Check sheet for the modelled part. Datum: model origin and axes. Units: mm. Give positions to 0.01 mm unless a question says otherwise; leave off trailing zeros. Order: outer loops, then holes, each group sorted by start corner. A loop starts at its lowest first (then second) coordinate and runs counter-clockwise, first axis right, second up.
```python
from build123d import *

# Parameters (mm, degrees)
ESQUISSE1_R        = 123.074849798
ESQUISSE1_R_2      = 2.953796395
ESQUISSE1_R_3      = 35
ESQUISSE1_R_4      = 3.375
ESQUISSE1_R_5      = 22.5
BOSS_EXTRU_1_DEPTH = 5
CHANFREIN1_SIZE    = 3


with BuildPart() as part:
    # Esquisse1 → Boss.-Extru.1 (new body)
    with BuildSketch(Plane.XY):
        Circle(ESQUISSE1_R)
        with Locations((0, 115.5)):
            Circle(ESQUISSE1_R_2, mode=Mode.SUBTRACT)
        Circle(ESQUISSE1_R_3, mode=Mode.SUBTRACT)
        with Locations((74.241968919, 88.47813318)):
            Circle(ESQUISSE1_R_2, mode=Mode.SUBTRACT)
        with Locations((113.745295473, 20.056364521)):
            Circle(ESQUISSE1_R_2, mode=Mode.SUBTRACT)
        with Locations((100.025934137, -57.75)):
            Circle(ESQUISSE1_R_2, mode=Mode.SUBTRACT)
        with Locations((39.503326554, -108.534497701)):
            Circle(ESQUISSE1_R_2, mode=Mode.SUBTRACT)
        with Locations((-39.503326554, -108.534497701)):
            Circle(ESQUISSE1_R_2, mode=Mode.SUBTRACT)
        with Locations((-100.025934137, -57.75)):
            Circle(ESQUISSE1_R_2, mode=Mode.SUBTRACT)
        with Locations((-113.745295473, 20.056364521)):
            Circle(ESQUISSE1_R_2, mode=Mode.SUBTRACT)
        with Locations((-74.241968919, 88.47813318)):
            Circle(ESQUISSE1_R_2, mode=Mode.SUBTRACT)
        with Locations((0, 50)):
            Circle(ESQUISSE1_R_4, mode=Mode.SUBTRACT)
        with Locations((50, 0)):
            Circle(ESQUISSE1_R_4, mode=Mode.SUBTRACT)
        with Locations((0, -50)):
            Circle(ESQUISSE1_R_4, mode=Mode.SUBTRACT)
        with Locations((-50, 0)):
            Circle(ESQUISSE1_R_4, mode=Mode.SUBTRACT)
        with Locations((0, 82.5)):
            Circle(ESQUISSE1_R_5, mode=Mode.SUBTRACT)
        with Locations((58.336309448, 58.336309448)):
            Circle(ESQUISSE1_R_5, mode=Mode.SUBTRACT)
        with Locations((82.5, 0)):
            Circle(ESQUISSE1_R_5, mode=Mode.SUBTRACT)
        with Locations((58.336309448, -58.336309448)):
            Circle(ESQUISSE1_R_5, mode=Mode.SUBTRACT)
        with Locations((0, -82.5)):
            Circle(ESQUISSE1_R_5, mode=Mode.SUBTRACT)
        with Locations((-58.336309448, -58.336309448)):
            Circle(ESQUISSE1_R_5, mode=Mode.SUBTRACT)
        with Locations((-82.5, 0)):
            Circle(ESQUISSE1_R_5, mode=Mode.SUBTRACT)
        with Locations((-58.336309448, 58.336309448)):
            Circle(ESQUISSE1_R_5, mode=Mode.SUBTRACT)
    extrude(amount=BOSS_EXTRU_1_DEPTH)

    # Chanfrein1
    chanfrein1_edges = [part.edges().sort_by_distance(p)[0] for p in [
        (71.288172524, 88.47813318, 0),
        (110.791499078, 20.056364521, 0),
        (97.072137742, -57.75, 0),
        (36.549530159, -108.534497701, 0),
        (-42.457122949, -108.534497701, 0),
        (-102.979730532, -57.75, 0),
        (-116.699091868, 20.056364521, 0),
        (-77.195765314, 88.47813318, 0),
        (-2.953796395, 115.5, 0),
    ]]
    chamfer(chanfrein1_edges, length=CHANFREIN1_SIZE)


solid = part.part
```
(1) Cross-section at A-A on x = -14. Enter the section's corners in (y, z).
Response values:
outline: (-122.28, 0) - (-100.11, 0) - (-100.11, 5) - (-122.28, 5) - close; (-64.89, 0) - (-32.08, 0) - (-32.08, 5) - (-64.89, 5) - close; (32.08, 0) - (64.89, 0) - (64.89, 5) - (32.08, 5) - close; (100.11, 0) - (122.28, 0) - (122.28, 5) - (100.11, 5) - close
(2) Gauge pin test, flat ends, axial feed: pin 1 Ø6 at (x, y) = (0, -50) entering from -Z; pin 2 Ø7.5 at (x, y) = (-39.5, -108.53) entering from -Z; pin 3 Ø3 at (y, z) = (-60.5, 1) entering from +X; pin 4 Ø3 at (y, z) = (-97.5, 1) entering from +X. Record the tip position at first contact, or that the pin passes through.
Response values:
pin 1: passes through
pin 2: stops at z = 2.2
pin 3: stops at x = 108.01
pin 4: stops at x = 77.02
(3) Cross-section at C-C on z = 1.2. Count the separate pieces of the cut face and the enclosed holes in it, then the cut area to 3 significant figures.
Response values:
separate pieces: 1
enclosed holes: 22
area: 30,200 mm2
(4) Cross-section at B-B on y = 115.5. Enter the section's corners in (x, z).
Response values:
outline: (-42.51, 0) - (-5.95, 0) - (-2.95, 3) - (-2.95, 5) - (-42.51, 5) - close; (2.95, 3) - (5.95, 0) - (42.51, 0) - (42.51, 5) - (2.95, 5) - close
(5) Material ranges on L1, parallel to X at y = 58.5, z = 4.65; L2, parallel to Y at x = -102.5, z = 1.35; L3, parallel to Y at x = -69.5, z = 3.3, recorded low to high.
Response values:
L1: x = -108.28 to -80.84, -35.84 to 35.84, 80.84 to 108.28
L2: y = -68.13 to -61.63, -53.87 to -10.31, 10.31 to 68.13
L3: y = -101.57 to -77.87, -38.8 to -18.36, 18.36 to 38.8, 77.87 to 101.57
(6) Release check for a two-part mould opening along Y. For faces 1 (the face through (26, -26, 0)), 2 (the face through (99.386, -60.634, 3.986)), 3 (the face through (103.022, -56.806, 2.812)) record: released by +Y, released by -Y, zero draft, split by the parting line, or undercut.
Response values:
face 1: zero draft
face 2: undercut
face 3: undercut
(7) Cross-section at D-D on y = 50. Enter the section's corners in (x, z) (3 decimals).
Response values:
outline: (-112.461, 0) - (-79.235, 0) - (-79.235, 5) - (-112.461, 5) - close; (-37.438, 0) - (-3.375, 0) - (-3.375, 5) - (-37.438, 5) - close; (3.375, 0) - (37.438, 0) - (37.438, 5) - (3.375, 5) - close; (79.235, 0) - (112.461, 0) - (112.461, 5) - (79.235, 5) - close
